from build123d import *

# Parameters (mm, degrees)
SKETCH1_R           = 50.8
BOSS_EXTRUDE1_DEPTH = 50.8
SKETCH2_R           = 31.75
BOSS_EXTRUDE2_DEPTH = 76.2
SKETCH3_W           = 98.373776994
SKETCH3_H           = 25.4
BOSS_EXTRUDE3_DEPTH = 63.5
SKETCH4_R           = 12.7
CUT_EXTRUDE1_DEPTH  = 151.804144505
FILLET1_R           = 25.4
FILLET2_R           = 25.4


with BuildPart() as part:
    # Sketch1 → Boss-Extrude1 (new body)
    with BuildSketch(Plane(origin=(0, 0, 0), x_dir=(1, 0, 0), z_dir=(0, 1, 0))):
        with Locations(Location((0, 0, 0), (0, 0, 270))):
            Circle(SKETCH1_R)
    extrude(amount=BOSS_EXTRUDE1_DEPTH)

    # Sketch2 → Boss-Extrude2 (add)
    with BuildSketch(Plane(origin=(0, 50.8, 0), x_dir=(1, 0, 0), z_dir=(0, 1, 0))):
        with Locations(Location((0, 0, 0), (0, 0, 90))):
            Circle(SKETCH2_R)
    extrude(amount=BOSS_EXTRUDE2_DEPTH)

    # Sketch3 → Boss-Extrude3 (add)
    with BuildSketch(Plane.XZ):
        Rectangle(SKETCH3_W, SKETCH3_H)
    extrude(amount=BOSS_EXTRUDE3_DEPTH)

    # Sketch4 → Cut-Extrude1 (cut, through all)
    with BuildSketch(Plane.XY.offset(12.7)):
        with Locations((0.243990196, -31.967064289)):
            Circle(SKETCH4_R)
    extrude(amount=-CUT_EXTRUDE1_DEPTH, mode=Mode.SUBTRACT)

    # Fillet1
    fillet1_edges = [part.edges().sort_by_distance(p)[0] for p in [
        (-49.186888497, -63.5, 0),
    ]]
    fillet(fillet1_edges, radius=FILLET1_R)

    # Fillet2
    fillet2_edges = [part.edges().sort_by_distance(p)[0] for p in [
        (49.186888497, -63.5, 0),
    ]]
    fillet(fillet2_edges, radius=FILLET2_R)


solid = part.part
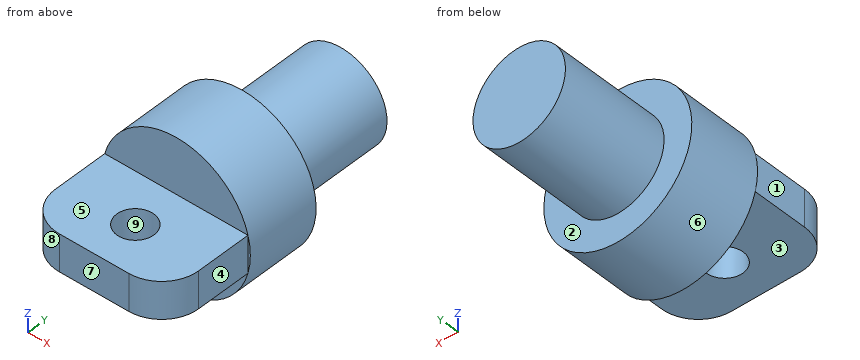
Build history of the part. All positions in model axes, mm. Face numbers are marked on the shaded views. A direction names the side the tool comes from. Give positions to 0.01 mm unless a question says otherwise; leave off trailing zeros. Order: outer loops, then holes, each group sorted by start corner. A loop starts at its lowest first (then second) coordinate and runs counter-clockwise, first axis right, second up. Notation, with made-up numbers: M 19,4.25 L 27,4.25 A29 cw 27,36.25 Z; hole C 82,-8 d8. An arc over 180 degrees is marked long. Use one line per item in the form item = value.
1) Drop flat-ended pins along their axis: pin 1 (8 mm diameter, centred on x = -36, z = -7, fed in from -Y); pin 2 (8 mm diameter, centred on x = -31, y = 71.5, fed in from -Z); pin 3 (11.5 mm diameter, centred on x = -19, z = 37.5, fed in from -Y). Give the stop position or say it passes through.
Calculated:
pin_1 = -62.14
pin_2 = -16.71
pin_3 = 0
2) Saw through at B-B (y = -21.5). Give the cut face in (x, z).
Calculated:
outline = M -49.19,-12.7 L -6.95,-12.7 L -6.95,12.7 L -49.19,12.7 Z; M 7.44,-12.7 L 49.19,-12.7 L 49.19,12.7 L 7.44,12.7 Z
3) Saw through at D-D (x = 36). Give the cut face in (y, z), plus the area to 3 significant figures.
Calculated:
outline = M -60.37,-12.7 L 0,-12.7 L 0,-35.84 L 50.8,-35.84 L 50.8,35.84 L 0,35.84 L 0,12.7 L -60.37,12.7 Z
area = 5,170 mm2
4) Tool access for the marked faces 1, 2, 3, 4 and 5: list every direction of +Z, -Z, +X, -X, +Y, -Y with a clear straight run to the whole face (end or side of a thin tool).
Calculated:
face_1 = +Z, -Z, -X, -Y
face_2 = +Y
face_3 = -Z, +X, -X, -Y
face_4 = +Z, -Z, +X, -Y
face_5 = +Z, +X, -X, -Y
5) Probe probe 1 along X at (y, z) = (-9.5, 2.5); probe 2 along Y at (x, z) = (17.5, -15); probe 3 along Y at (x, z) = (17.5, 28.5). List the from-to ranges inside material, lowest first.
Calculated:
probe_1 = -49.19 to 49.19
probe_2 = 0 to 127
probe_3 = 0 to 50.8
6) Saw through at A-A (x = 0). Give the cut face in (y, z), plus the area to 3 significant figures.
Calculated:
outline = M -63.5,-12.7 L -44.66,-12.7 L -44.66,12.7 L -63.5,12.7 Z; M -19.27,-12.7 L 0,-12.7 L 0,-50.8 L 50.8,-50.8 L 50.8,-31.75 L 127,-31.75 L 127,31.75 L 50.8,31.75 L 50.8,50.8 L 0,50.8 L 0,12.7 L -19.27,12.7 Z
area = 11,000 mm2
7) Two-plate mould, pull along X, no slides. Class the marked faces 6, 7, 8 and 9: released by +X, released by -X, zero draft, split by the parting line, or undercut.
Calculated:
face_6 = split by the parting line
face_7 = zero draft
face_8 = released by -X
face_9 = undercut
8) Saw through at C-C (z = 9). Give the cut face in (x, y).
Calculated:
outline = M -50,0 L -49.19,0 L -49.19,-38.1 A25.4 ccw -23.79,-63.5 L 23.79,-63.5 A25.4 ccw 49.19,-38.1 L 49.19,0 L 50,0 L 50,50.8 L 30.45,50.8 L 30.45,127 L -30.45,127 L -30.45,50.8 L -50,50.8 Z; hole C 0.24,-31.97 d25.4
